The listing builds one solid part. Answer for the finished solid, in the listing's coordinates (mm). Face numbers are marked on the shaded views. A direction names the side the tool comes from. Give positions to 0.01 mm unless a question says otherwise; leave off trailing zeros. Write each loop counter-clockwise with the first axis right and the second up, starting at its lowest first coordinate (ties: lowest second). Pieces come first, ordered by that corner, then holes. Notation, with made-up numbers: (8, 40) -> (16, 40) arc R16 cw to (16, 50) -> close; hole circle Ø5 at (37, -2.75). An arc over 180 degrees is marked (long way). Put each result on its own line as item: value. Start each with the question number.
1) A cutting plane is placed at A-A (y = -31). Write down the section's boundary in (x, z), then the cut area to 3 significant figures.
2) Find the intervals of material crossed by line 1 along X through (y, z) = (-27, 9.5); line 2 along Y through (x, z) = (24, -26); line 3 along Z through (x, y) = (19.5, -31), in increasing order. Write a range as from..to.
3) For a pull along X with two mould halves and no side action, classify the marked faces 6, 7 and 8 as released by +X, released by -X, zero draft, split by the parting line, or undercut.
4) For the marked faces 1, 2, 3, 4 and 5, determine the directions among +Z, -Z, +X, -X, +Y, -Y from which every point of the face is accessible in a straight line to the end or side of a thin tool.
5) A cutting plane is placed at C-C (z = -26). Write down the section's boundary in (x, y).
6) A cutting plane is placed at D-D (y = -14.5). Write down the section's boundary in (x, z), then the cut area to 3 significant figures.
7) A cutting plane is placed at B-B (x = -10). Write down the section's boundary in (y, z), then the cut area to 3 significant figures.
8) Flat-ended cylindrical pins translate along their axes: pin 1 Ø12 at (x, y) = (-8.5, -32) entering from +Z; pin 2 Ø20 at (x, y) = (-0.5, -32.5) entering from -Z; pin 3 Ø10 at (y, z) = (-31.5, 2.5) entering from -X. Find the tip coordinate at first contact, or state that the pin passes through.
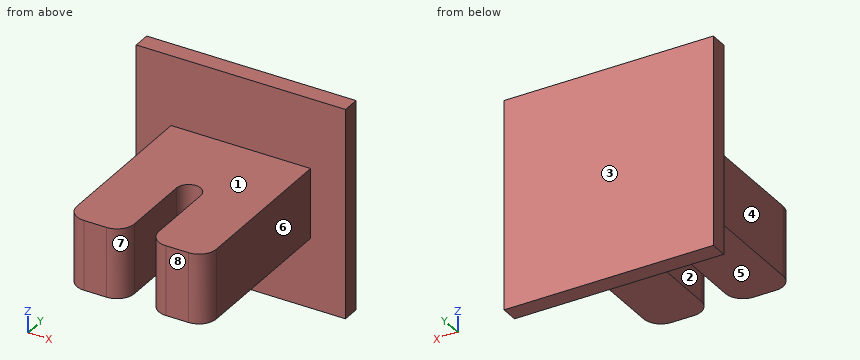
from build123d import *

# Parameters (mm, degrees)
F1_DEPTH = 50
F3_DEPTH = 25
F5_DEPTH = 5
F6_R     = 5


with BuildPart() as f1:
    # F0 (on Front) → F1 (new body)
    with BuildSketch(Plane.XZ):
        Polygon((20, 10), (0, 10), (-20, 10), (-20, -10), (20, -10), align=None)
    extrude(amount=F1_DEPTH)

    # F2 (on face) → F3 (cut)
    with BuildSketch(Plane(origin=(0, 0, -10), x_dir=(1, 0, 0), z_dir=(0, 0, -1))):
        with BuildLine():
            Line((-3.5, 50), (-3.5, 25))
            ThreePointArc((-3.5, 25), (0, 21.5), (3.5, 25))
            Line((3.5, 25), (3.5, 50))
            Line((3.5, 50), (-3.5, 50))
        make_face()
    extrude(amount=-F3_DEPTH, mode=Mode.SUBTRACT)

    # F4 (on face) → F5 (join)
    with BuildSketch(Plane(origin=(0, 0, 0), x_dir=(-1, 0, 0), z_dir=(0, 1, 0))):
        Polygon((-30, 30), (-30, 0), (-30, -30), (30, -30), (30, 30), align=None)
        Polygon((-20, -10), (-20, 0), (-20, 10), (20, 10), (20, -10), align=None, mode=Mode.SUBTRACT)
        Polygon((-20, 10), (-20, 0), (-20, -10), (20, -10), (20, 10), align=None)
    extrude(amount=F5_DEPTH)

    # F6
    f6_edges = [f1.edges().sort_by_distance(p)[0] for p in [
        (20, -50, 0),
        (3.5, -50, 0),
        (-3.5, -50, 0),
        (-20, -50, 0),
    ]]
    fillet(f6_edges, radius=F6_R)


solid = f1.part
Reply:
1. outline: (-20, -10) -> (-3.5, -10) -> (-3.5, 10) -> (-20, 10) -> close; (3.5, -10) -> (20, -10) -> (20, 10) -> (3.5, 10) -> close
1. area: 660 mm2
2. line 1: x = -20..-3.5, 3.5..20
2. line 2: y = 0..5
2. line 3: z = -10..10
3. face 6: released by +X
3. face 7: undercut
3. face 8: zero draft
4. face 1: +Z, +X, -X, -Y
4. face 2: +Z, -Z, -Y
4. face 3: +Z, -Z, +X, -X, +Y
4. face 4: +Z, -Z, -X, -Y
4. face 5: -Z, +X, -X, -Y
5. outline: (-30, 0) -> (30, 0) -> (30, 5) -> (-30, 5) -> close
6. outline: (-20, -10) -> (20, -10) -> (20, 10) -> (-20, 10) -> close
6. area: 800 mm2
7. outline: (-50, -10) -> (0, -10) -> (0, -30) -> (5, -30) -> (5, 30) -> (0, 30) -> (0, 10) -> (-50, 10) -> close
7. area: 1,300 mm2
8. pin 1: stops at z = 10
8. pin 2: stops at z = -10
8. pin 3: stops at x = -20
